Here's how the part is built. I have some questions about the finished solid (model axes, mm). Face numbers are marked on the shaded views. A direction names the side the tool comes from. Coordinates: 2 decimals unless noted, no trailing zeros. Write each loop counter-clockwise with the first axis right and the second up, starting at its lowest first coordinate (ties: lowest second). Pieces come first, ordered by that corner, then holes. Notation, with made-up numbers: (43.5, 83) -> (60.5, 83) arc R20 cw to (60.5, 90) -> close; hole circle Ø4 at (65, 68.25). An arc over 180 degrees is marked (long way). Put each result on its own line as item: value.
```python
from build123d import *

# Parameters (mm, degrees)
SKETCH_1_W          = 60
SKETCH_1_H          = 37
SKETCH_1_R          = 1.5
EXTRUDE_1_DEPTH     = 1
SKETCH_2_W          = 18
SKETCH_2_H          = 20
EXTRUDE_2_DEPTH     = 10
SKETCH_3_R          = 1
CUT_EXTRUDE_1_DEPTH = 1
SKETCH_4_W          = 1.889309118
SKETCH_4_H          = 3.828785833
CUT_EXTRUDE_2_DEPTH = 5
SKETCH_5_W          = 6
SKETCH_5_H          = 17
EXTRUDE_3_DEPTH     = 7
SKETCH_6_W          = 4.219200818
SKETCH_6_H          = 14.571651166
CUT_EXTRUDE_3_DEPTH = 7
SKETCH_7_W          = 1.099481737
SKETCH_7_H          = 10
EXTRUDE_4_DEPTH     = 17
SKETCH_8_W          = 3
SKETCH_8_H          = 10
EXTRUDE_5_DEPTH     = 9
SKETCH_9_R          = 1.5
CUT_EXTRUDE_4_DEPTH = 9
SKETCH_10_W         = 8.015050441
SKETCH_10_H         = 8.015050442
SKETCH_10_W_2       = 5.788647541
SKETCH_10_H_2       = 13.284723362
EXTRUDE_7_DEPTH     = 5
SKETCH_11_R         = 4.452805801
EXTRUDE_8_DEPTH     = 12
SKETCH_12_W         = 40
SKETCH_12_H         = 37
EXTRUDE_9_DEPTH     = 10
SKETCH_13_W         = 2.63
SKETCH_13_H         = 7.995738943
CUT_EXTRUDE_5_DEPTH = 64.941379403
SKETCH_14_W         = 11
SKETCH_14_H         = 20
CUT_EXTRUDE_6_DEPTH = 49.448426187


with BuildPart() as part:
    # 草图1 → 凸台-拉伸1 (new body)
    with BuildSketch(Plane(origin=(0, 0, 0), x_dir=(1, 0, 0), z_dir=(0, 1, 0))):
        Rectangle(SKETCH_1_W, SKETCH_1_H)
        with Locations(Location((27, 15, 0), (0, 0, 270))):
            Circle(SKETCH_1_R, mode=Mode.SUBTRACT)
        with Locations(Location((27, -15, 0), (0, 0, 90))):
            Circle(SKETCH_1_R, mode=Mode.SUBTRACT)
        with Locations(Location((-27, -15, 0), (0, 0, 270))):
            Circle(SKETCH_1_R, mode=Mode.SUBTRACT)
        with Locations(Location((-27, 15, 0), (0, 0, 90))):
            Circle(SKETCH_1_R, mode=Mode.SUBTRACT)
    extrude(amount=EXTRUDE_1_DEPTH)

    # 草图2 → 凸台-拉伸2 (add)
    with BuildSketch(Plane(origin=(0, 1, 0), x_dir=(1, 0, 0), z_dir=(0, 1, 0))):
        with Locations((32, 0)):
            Rectangle(SKETCH_2_W, SKETCH_2_H)
    extrude(amount=EXTRUDE_2_DEPTH)

    # 草图3 → 切除-拉伸1 (cut)
    with BuildSketch(Plane(origin=(0, 11, 0), x_dir=(1, 0, 0), z_dir=(0, 1, 0))):
        with Locations(Location((38.562083072, 7.5, 0), (0, 0, 270))):
            Circle(SKETCH_3_R)
        with Locations(Location((38.562083072, 2.5, 0), (0, 0, 270))):
            Circle(SKETCH_3_R)
        with Locations(Location((38.562083072, -7.5, 0), (0, 0, 90))):
            Circle(SKETCH_3_R)
        with Locations(Location((38.562083072, -2.5, 0), (0, 0, 90))):
            Circle(SKETCH_3_R)
    extrude(amount=-CUT_EXTRUDE_1_DEPTH, mode=Mode.SUBTRACT)

    # 草图4 → 切除-拉伸2 (cut)
    with BuildSketch(Plane(origin=(41, 0, 0), x_dir=(0, 0, -1), z_dir=(1, 0, 0))):
        with Locations((-2.5, 3.73063685)):
            Rectangle(SKETCH_4_W, SKETCH_4_H)
        with Locations((-7.5, 3.73063685)):
            Rectangle(SKETCH_4_W, SKETCH_4_H)
        with Locations((2.5, 3.73063685)):
            Rectangle(SKETCH_4_W, SKETCH_4_H)
        with Locations((7.5, 3.73063685)):
            Rectangle(SKETCH_4_W, SKETCH_4_H)
    extrude(amount=-CUT_EXTRUDE_2_DEPTH, mode=Mode.SUBTRACT)

    # 草图5 → 凸台-拉伸3 (add)
    with BuildSketch(Plane(origin=(0, 1, 0), x_dir=(1, 0, 0), z_dir=(0, 1, 0))):
        with Locations((-27, 3)):
            Rectangle(SKETCH_5_W, SKETCH_5_H)
    extrude(amount=EXTRUDE_3_DEPTH)

    # 草图6 → 切除-拉伸3 (cut)
    with BuildSketch(Plane(origin=(0, 8, 0), x_dir=(1, 0, 0), z_dir=(0, 1, 0))):
        with Locations((-27, 3)):
            Rectangle(SKETCH_6_W, SKETCH_6_H)
    extrude(amount=-CUT_EXTRUDE_3_DEPTH, mode=Mode.SUBTRACT)

    # 草图7 → 凸台-拉伸4 (add)
    with BuildSketch(Plane(origin=(0, 1, 0), x_dir=(1, 0, 0), z_dir=(0, 1, 0))):
        with Locations((-23.450259132, -13.5)):
            Rectangle(SKETCH_7_W, SKETCH_7_H)
    extrude(amount=EXTRUDE_4_DEPTH)

    # 草图8 → 凸台-拉伸5 (add)
    with BuildSketch(Plane(origin=(0, 1, 0), x_dir=(1, 0, 0), z_dir=(0, 1, 0))):
        with Locations((-21.400518263, -13.5)):
            Rectangle(SKETCH_8_W, SKETCH_8_H)
    extrude(amount=EXTRUDE_5_DEPTH)

    # 草图9 → 切除-拉伸4 (cut)
    with BuildSketch(Plane(origin=(-22.900518263, 0, 0), x_dir=(0, 0, -1), z_dir=(1, 0, 0))):
        with Locations((-13.5, 14.366101357)):
            Circle(SKETCH_9_R)
    extrude(amount=-CUT_EXTRUDE_4_DEPTH, mode=Mode.SUBTRACT)

    # 草图10 → 凸台-拉伸7 (add)
    with BuildSketch(Plane(origin=(0, 1, 0), x_dir=(1, 0, 0), z_dir=(0, 1, 0))):
        with Locations((2.23408969, 2.63483646)):
            Rectangle(SKETCH_10_W, SKETCH_10_H)
        with Locations((-16.318748425, 6.642361681)):
            Rectangle(SKETCH_10_W_2, SKETCH_10_H_2)
        with Locations((17.76591031, 2.63483646)):
            Rectangle(SKETCH_10_W, SKETCH_10_H)
        with Locations((17.76591031, -11.63483646)):
            Rectangle(SKETCH_10_W, SKETCH_10_H)
        with Locations((2.23408969, -11.63483646)):
            Rectangle(SKETCH_10_W, SKETCH_10_H)
    extrude(amount=EXTRUDE_7_DEPTH)

    # 草图11 → 凸台-拉伸8 (add)
    with BuildSketch(Plane(origin=(0, 1, 0), x_dir=(1, 0, 0), z_dir=(0, 1, 0))):
        with Locations(Location((-11.643302333, -10.85371414, 0), (0, 0, 270))):
            Circle(SKETCH_11_R)
    extrude(amount=EXTRUDE_8_DEPTH)

    # 草图12 → 凸台-拉伸9 (add)
    with BuildSketch(Plane.XZ):
        with Locations((2.5, 0)):
            Rectangle(SKETCH_12_W, SKETCH_12_H)
    extrude(amount=EXTRUDE_9_DEPTH)

    # 草图13 → 切除-拉伸5 (cut, through all)
    with BuildSketch(Plane.ZY.offset(17.5)):
        with Locations((-16.185, -6.002130529)):
            Rectangle(SKETCH_13_W, SKETCH_13_H)
        with Locations((-11.565, -6.002130529)):
            Rectangle(SKETCH_13_W, SKETCH_13_H)
        with Locations((-6.935, -6.002130529)):
            Rectangle(SKETCH_13_W, SKETCH_13_H)
        with Locations((-2.315, -6.002130529)):
            Rectangle(SKETCH_13_W, SKETCH_13_H)
        with Locations((2.315, -6.002130529)):
            Rectangle(SKETCH_13_W, SKETCH_13_H)
        with Locations((6.935, -6.002130529)):
            Rectangle(SKETCH_13_W, SKETCH_13_H)
        with Locations((11.565, -6.002130529)):
            Rectangle(SKETCH_13_W, SKETCH_13_H)
        with Locations((16.185, -6.002130529)):
            Rectangle(SKETCH_13_W, SKETCH_13_H)
    extrude(amount=-CUT_EXTRUDE_5_DEPTH, mode=Mode.SUBTRACT)

    # 草图14 → 切除-拉伸6 (cut, through all)
    with BuildSketch(Plane.XZ):
        with Locations((35.5, 0)):
            Rectangle(SKETCH_14_W, SKETCH_14_H)
    extrude(amount=-CUT_EXTRUDE_6_DEPTH, mode=Mode.SUBTRACT)


solid = part.part
```
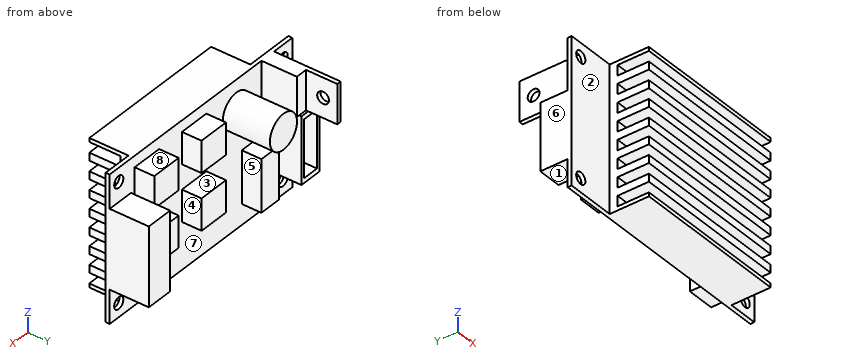
Item 1: Imagine slicing it at D-D on x = 27. Write out the boundary of the cut face in (y, z), then the cut area to 3 significant figures.
Output:
outline: (0, -18.5) -> (1, -18.5) -> (1, -16.5) -> (0, -16.5) -> close; (0, -13.5) -> (1, -13.5) -> (1, -10) -> (11, -10) -> (11, 10) -> (1, 10) -> (1, 13.5) -> (0, 13.5) -> close; (0, 16.5) -> (1, 16.5) -> (1, 18.5) -> (0, 18.5) -> close
area: 231 mm²
Item 2: Imagine slicing it at C-C on y = -1. Write out the boundary of the cut face in (x, z).
Output:
outline: (-17.5, -18.5) -> (22.5, -18.5) -> (22.5, 18.5) -> (-17.5, 18.5) -> close
Item 3: Please list where these lines run through material, in increasing order: line 1 along X through (y, z) = (0.25, 15); line 2 along X through (y, z) = (7.5, 3); line 3 along Y through (x, z) = (-23.3, 13.5). Write a range as from..to.
Output:
line 1: x = -30..-28.5, -25.5..25.5, 28.5..30
line 2: x = -30..-29.11, -24.89..-24, 23..30
line 3: y = 0..12.87, 15.87..18
Item 4: Imagine slicing it at B-B on z = -7.5. Write out the boundary of the cut face in (x, y).
Output:
outline: (-30, 0) -> (-17.5, 0) -> (-17.5, -2) -> (22.5, -2) -> (22.5, 0) -> (30, 0) -> (30, 11) -> (23, 11) -> (23, 1) -> (-13.42, 1) -> (-13.42, 6) -> (-19.21, 6) -> (-19.21, 1) -> (-24, 1) -> (-24, 8) -> (-24.89, 8) -> (-24.89, 1) -> (-29.11, 1) -> (-29.11, 8) -> (-30, 8) -> close
Item 5: For P1, Ø10, axis at x = -20, z = 2, coming from the -Y side; P2, Ø6, axis at x = -7.5, y = 9.5, coming from the +Z side; P3, Ø1.5, axis at x = 19, y = 4, coming from the +Z side; P4, Ø0.9, axis at x = -22, z = 12.5, coming from the +Y side, each with a flat end and sliding along its axis, tell me the tip position at first contact or that it passes through.
Output:
P1: stops at y = -10
P2: stops at z = 15.16
P3: stops at z = 15.64
P4: stops at y = 10
Item 6: Which directions (+Z, -Z, +X, -X, +Y, -Y) give clear straight access to the entire face, cutting with the end or side of a thin tool? Please do the marked faces 1, 2, 3, 4 and 5.
Output:
face 1: -Z, -X, +Y
face 2: +Z, -Z, -X, -Y
face 3: +Y
face 4: +Z, -Z, +Y
face 5: -Z, +Y
Item 7: Imagine slicing it at A-A on x = -27. Write out the boundary of the cut face in (y, z), then the cut area to 3 significant figures.
Output:
outline: (0, -18.5) -> (1, -18.5) -> (1, -16.5) -> (0, -16.5) -> close; (0, -13.5) -> (1, -13.5) -> (1, -11.5) -> (8, -11.5) -> (8, -10.29) -> (1, -10.29) -> (1, 4.29) -> (8, 4.29) -> (8, 5.5) -> (1, 5.5) -> (1, 13.5) -> (0, 13.5) -> close; (0, 16.5) -> (1, 16.5) -> (1, 18.5) -> (0, 18.5) -> close
area: 48.0 mm²
Item 8: If we mould it in two halves opening along X, with no side actions, what happens to the marked faces 6, 7 and 8? For each: released by +X, released by -X, zero draft, split by the parting line, or undercut.
Output:
face 6: released by -X
face 7: undercut
face 8: zero draft
